Input: part model. Units: mm. Frame: model coordinates. Face numbers are marked on the shaded views. A direction names the side the tool comes from. Coordinates: 2 decimals unless noted, no trailing zeros. Loops run counter-clockwise (first coordinate to the right, second up) from the corner with the lowest first, then second, coordinate; pieces in that order, holes last. Notation, with made-up numbers: (36.5, 74) -> (50.5, 74) arc R29 ccw to (50.5, 109) -> close; hole circle Ø9 at (55.5, -2). An arc over 180 degrees is marked (long way). Answer as a JSON object with one key per item and string values.
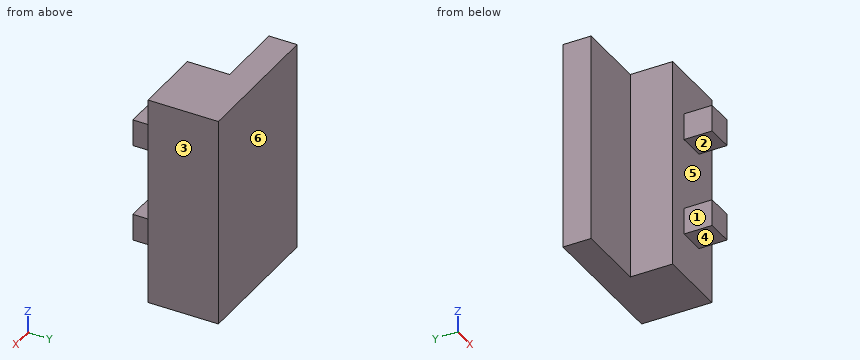
Autodesk Inventor part; units mm, degrees
ref_plane "YZ Plane" through (0, 0, 0) normal (1, 0, 0) x (0, 1, 0)
ref_plane "XZ Plane" through (0, 0, 0) normal (0, 1, 0) x (-1, 0, 0)
ref_plane "XY Plane" through (0, 0, 0) normal (0, 0, 1) x (1, 0, 0)
sketch "Sketch1" plane through (0, 0, 0) normal (0, 1, 0) x (-1, 0, 0)
  line L0 (-5, 7.5) -> (5, 7.5)
  line L1 (5, 7.5) -> (5, -7.5)
  line L2 (5, -7.5) -> (-5, -7.5)
  line L3 (-5, -7.5) -> (-5, 7.5)
  line L4 (-5, 7.5) -> (5, -7.5) construction
  line L5 (5, 7.5) -> (-5, -7.5) construction
  point P0 (0, 0)
  dimension "d0" = 10
  dimension "d1" = 15
extrude "Extrusion1" add sketch "Sketch1" along normal mid plane 5
sketch "Sketch2" plane through (-5, 2.5, 7.5) normal (0, 0, 1) x (1, 0, 0)
  line L0 (0, 0) -> (0, -5)
  line L1 (5, -2) -> (0, -2)
  line L2 (0, -2) -> (0, -5)
  line L3 (0, -5) -> (5, -5)
  line L4 (5, -5) -> (5, -2)
  line L5 (5, -2) -> (0, -5) construction
  line L6 (0, -2) -> (5, -5) construction
  point P0 (5, -2.5)
  point P1 (2.5, -3.5)
  dimension "d4" = 5
  dimension "d13" = 3
extrude "Extrusion2" cut sketch "Sketch2" against normal through all
sketch "Sketch3" plane through (0, -2.5, 0) normal (0, -1, 0) x (1, 0, 0)
  line L0 (3.4, 4.5) -> (1.4, 4.5) construction
  line L1 (1.4, 4.5) -> (1.4, 2.5) construction
  line L2 (1.4, 2.5) -> (3.4, 2.5) construction
  line L3 (3.4, 2.5) -> (3.4, 4.5) construction
  line L4 (3.4, 4.5) -> (1.4, 2.5) construction
  line L5 (1.4, 4.5) -> (3.4, 2.5) construction
  line L6 (3.4, -2.5) -> (1.4, -2.5) construction
  line L7 (1.4, -2.5) -> (1.4, -4.5) construction
  line L8 (1.4, -4.5) -> (3.4, -4.5) construction
  line L9 (3.4, -4.5) -> (3.4, -2.5) construction
  line L10 (3.4, -2.5) -> (1.4, -4.5) construction
  line L11 (1.4, -2.5) -> (3.4, -4.5) construction
  line L12 (2.4, 3.5) -> (2.4, -3.5) construction
  line L13 (3.35, 2.55) -> (1.45, 2.55)
  line L14 (1.45, 2.55) -> (1.45, 4.45)
  line L15 (1.45, 4.45) -> (3.35, 4.45)
  line L16 (3.35, 4.45) -> (3.35, 2.55)
  line L17 (1.45, -2.55) -> (3.35, -2.55)
  line L18 (3.35, -2.55) -> (3.35, -4.45)
  line L19 (3.35, -4.45) -> (1.45, -4.45)
  line L20 (1.45, -4.45) -> (1.45, -2.55)
  line L21 (5, -7.5) -> (5, 7.5)
  point P0 (0, 0)
  point P1 (2.4, 0)
  dimension "d7" = 2
  dimension "d8" = 7
  dimension "d11" = 0.05
  dimension "d12" = 0.05
  dimension "d14" = 2.6
extrude "Extrusion3" add sketch "Sketch3" along normal blind 2
properties part number "AlignmentPiece"
1. Line query: line 1 along Y through (x, z) = (-0.25, -4.75); line 2 along X through (y, z) = (-2, -3.75); line 3 along Y through (x, z) = (2.75, -4.5). Output: solid intervals per line, ascending.
Reply:
{"line 1": "y = 0.5 to 2.5", "line 2": "x = 0 to 5", "line 3": "y = -2.5 to 2.5"}
2. Section query C-C (x = -2). Return loops of the section in (y, z).
Reply:
{"outline": "(0.5, -7.5) -> (2.5, -7.5) -> (2.5, 7.5) -> (0.5, 7.5) -> close"}
3. Pin query (flat end, axial travel): P1, Ø1.5, axis at x = 3.5, z = -3, coming from the -Y side; P2, Ø1.5, axis at y = -3.5, z = 3, coming from the +X side; P3, Ø3.5, axis at y = -1.5, z = 2, coming from the -X side; P4, Ø1.5, axis at x = -2, z = -1, coming from the -Y side. Return the tip coordinate at first contact, or that it passes through.
Reply:
{"P1": "stops at y = -4.5", "P2": "stops at x = 3.35", "P3": "stops at x = 0", "P4": "stops at y = 0.5"}
4. Access query for the marked faces 1, 2 and 3. Directions: +Z, -Z, +X, -X, +Y, -Y. A direction counts if a zero-diameter tool reaches every point of the face in a straight line with its end or side. Return the directions, or none.
Reply:
{"face 1": "+Z, -Z, -X, -Y", "face 2": "+X, -X, -Y", "face 3": "+Z, -Z, +X, +Y, -Y"}
5. Section query D-D (y = -2). Return loops of the section in (x, z).
Reply:
{"outline": "(0, -7.5) -> (5, -7.5) -> (5, 7.5) -> (0, 7.5) -> close"}
6. Section query A-A (y = -4). Return loops of the section in (x, z), plus the area to 3 significant figures.
Reply:
{"outline": "(1.45, -4.45) -> (3.35, -4.45) -> (3.35, -2.55) -> (1.45, -2.55) -> close; (1.45, 2.55) -> (3.35, 2.55) -> (3.35, 4.45) -> (1.45, 4.45) -> close", "area": "7.22 mm2"}
7. Section query B-B (z = 4.75). Return loops of the section in (x, y).
Reply:
{"outline": "(-5, 0.5) -> (0, 0.5) -> (0, -2.5) -> (5, -2.5) -> (5, 2.5) -> (-5, 2.5) -> close"}
8. Mould query, pull axis Z, two halves, no side actions, for the marked faces 4, 5 and 6. Classes: pulls with the +Z half, pulls with the -Z half, needs draft (parallel to the pull), parting line crosses it, or undercut.
Reply:
{"face 4": "pulls with the -Z half", "face 5": "undercut", "face 6": "needs draft"}
